```python
from build123d import *

# Parameters (mm, degrees)
SKETCH1_W           = 121
SKETCH1_H           = 66
BOSS_EXTRUDE1_DEPTH = 3.8
SKETCH2_W           = 109
SKETCH2_H           = 58
CUT_EXTRUDE1_DEPTH  = 138.881978518
FILLET1_R           = 5
SKETCH3_W           = 20
SKETCH3_H           = 58
BOSS_EXTRUDE2_DEPTH = 3.8
FILLET2_R           = 3
SKETCH4_R           = 1
CUT_EXTRUDE2_DEPTH  = 138.881978518
BOSS_EXTRUDE3_DEPTH = 3.8
SKETCH6_R           = 1.75
CUT_EXTRUDE3_DEPTH  = 156.841072892
FILLET3_R           = 5


with BuildPart() as part:
    # Sketch1 → Boss-Extrude1 (new body)
    with BuildSketch(Plane(origin=(0, 0, 0), x_dir=(1, 0, 0), z_dir=(0, 1, 0))):
        with Locations((60.5, -33)):
            Rectangle(SKETCH1_W, SKETCH1_H)
    extrude(amount=BOSS_EXTRUDE1_DEPTH)

    # Sketch2 → Cut-Extrude1 (cut, through all)
    with BuildSketch(Plane(origin=(0, 3.8, 0), x_dir=(1, 0, 0), z_dir=(0, 1, 0))):
        with Locations((60.5, -33)):
            Rectangle(SKETCH2_W, SKETCH2_H)
    extrude(amount=-CUT_EXTRUDE1_DEPTH, mode=Mode.SUBTRACT)

    # Fillet1
    fillet1_edges = [part.edges().sort_by_distance(p)[0] for p in [
        (115, 1.9, 4),
        (115, 1.9, 62),
        (6, 1.9, 62),
        (6, 1.9, 4),
    ]]
    fillet(fillet1_edges, radius=FILLET1_R)

    # Sketch3 → Boss-Extrude2 (add, through all)
    with BuildSketch(Plane(origin=(0, 3.8, 0), x_dir=(1, 0, 0), z_dir=(0, 1, 0))):
        with Locations((60.5, -33)):
            Rectangle(SKETCH3_W, SKETCH3_H)
    extrude(amount=-BOSS_EXTRUDE2_DEPTH)

    # Fillet2
    fillet2_edges = [part.edges().sort_by_distance(p)[0] for p in [
        (70.5, 1.9, 4),
        (70.5, 1.9, 62),
        (50.5, 1.9, 62),
        (50.5, 1.9, 4),
    ]]
    fillet(fillet2_edges, radius=FILLET2_R)

    # Sketch4 → Cut-Extrude2 (cut, through all)
    with BuildSketch(Plane(origin=(0, 3.8, 0), x_dir=(1, 0, 0), z_dir=(0, 1, 0))):
        with Locations(Location((116.5, -61.5, 0), (0, 0, 270))):
            Circle(SKETCH4_R)
        with Locations(Location((116.5, -4.5, 0), (0, 0, 270))):
            Circle(SKETCH4_R)
        with Locations(Location((4.5, -4.5, 0), (0, 0, 270))):
            Circle(SKETCH4_R)
        with Locations(Location((4.5, -61.5, 0), (0, 0, 270))):
            Circle(SKETCH4_R)
    extrude(amount=-CUT_EXTRUDE2_DEPTH, mode=Mode.SUBTRACT)

    # Sketch5 → Boss-Extrude3 (add, through all)
    with BuildSketch(Plane(origin=(0, 3.8, 0), x_dir=(1, 0, 0), z_dir=(0, 1, 0))):
        Polygon((0, 0), (-15, 0), (-15, -76), (136, -76), (136, 0), (121, 0), (121, -66), (0, -66), align=None)
    extrude(amount=-BOSS_EXTRUDE3_DEPTH)

    # Sketch6 → Cut-Extrude3 (cut, through all)
    with BuildSketch(Plane(origin=(0, 0, 0), x_dir=(-1, 0, 0), z_dir=(0, -1, 0))):
        with Locations(Location((10, -71, 0), (0, 0, 90))):
            Circle(SKETCH6_R)
        with Locations(Location((10, -5, 0), (0, 0, 90))):
            Circle(SKETCH6_R)
        with Locations(Location((-131, -71, 0), (0, 0, 90))):
            Circle(SKETCH6_R)
        with Locations(Location((-131, -5, 0), (0, 0, 90))):
            Circle(SKETCH6_R)
    extrude(amount=-CUT_EXTRUDE3_DEPTH, mode=Mode.SUBTRACT)

    # Fillet3
    fillet3_edges = [part.edges().sort_by_distance(p)[0] for p in [
        (136, 1.9, 0),
        (136, 1.9, 76),
        (-15, 1.9, 76),
        (-15, 1.9, 0),
    ]]
    fillet(fillet3_edges, radius=FILLET3_R)


solid = part.part
```
Source: CAD feature listing. Evaluate the final solid. Frame: model axes, mm. A direction names the side the tool comes from. Coordinates: 2 decimals unless noted, no trailing zeros. Order: outer loops, then holes, each group sorted by start corner. A loop starts at its lowest first (then second) coordinate and runs counter-clockwise, first axis right, second up. Notation, with made-up numbers: (-18, 65.25) - (14, 65.25) arc R17 ccw to (14, 98.25) - close; hole circle Ø7 at (38, 27). An arc over 180 degrees is marked (long way). One line per item, written item: value.
1) Mould query, pull axis X, two halves, no side actions, for faces 1 (the face through (-13, 2, 1)), 2 (the face through (134, 2, 1)), 3 (the face through (8, 2, 61)), 4 (the face through (59, 3.8, 37)). Classes: released by +X, released by -X, zero draft, split by the parting line, or undercut.
Computed values:
face 1: released by -X
face 2: released by +X
face 3: undercut
face 4: zero draft
2) Contact query for a flat-ended pin moving along its axis: pin 1 (3 mm diameter, centred on x = 116.5, z = 4.5, fed in from -Y). Output: stop coordinate, or through.
Computed values:
pin 1: stops at y = 0
3) Cut plane A-A on x = 34. Output: boundary loops of the cut face in (y, z).
Computed values:
outline: (0, 0) - (3.8, 0) - (3.8, 4) - (0, 4) - close; (0, 62) - (3.8, 62) - (3.8, 76) - (0, 76) - close
4) Cut plane C-C on z = 12.5. Output: boundary loops of the cut face in (x, y).
Computed values:
outline: (-15, 0) - (6, 0) - (6, 3.8) - (-15, 3.8) - close; (50.5, 0) - (70.5, 0) - (70.5, 3.8) - (50.5, 3.8) - close; (115, 0) - (136, 0) - (136, 3.8) - (115, 3.8) - close
5) Reachability of faces 5 (the face through (-14, 2, 74)), 6 (the face through (8, 2, 5)) from +Z, -Z, +X, -X, +Y, -Y: full face, straight path, thin tool, end or side. Return the list, or none.
Computed values:
face 5: +Z, -X, +Y, -Y
face 6: +Y, -Y
6) Cut plane B-B on y = 3.1. State how many separate pieces and enclosed holes the cut face has, plus the area to 3 significant figures.
Computed values:
separate pieces: 1
enclosed holes: 10
area: 6,270 mm^2
7) Ray query, line 1 (X direction, y = 2.1, z = 41.5); line 2 (Z direction, x = 131, y = 2.25); line 3 (Z direction, x = 79, y = 3.65). Return the intervals inside material, ascending. Write a range as [from, to].
Computed values:
line 1: x = [-15, 6], [50.5, 70.5], [115, 136]
line 2: z = [0, 3.25], [6.75, 69.25], [72.75, 76]
line 3: z = [0, 4], [62, 76]
